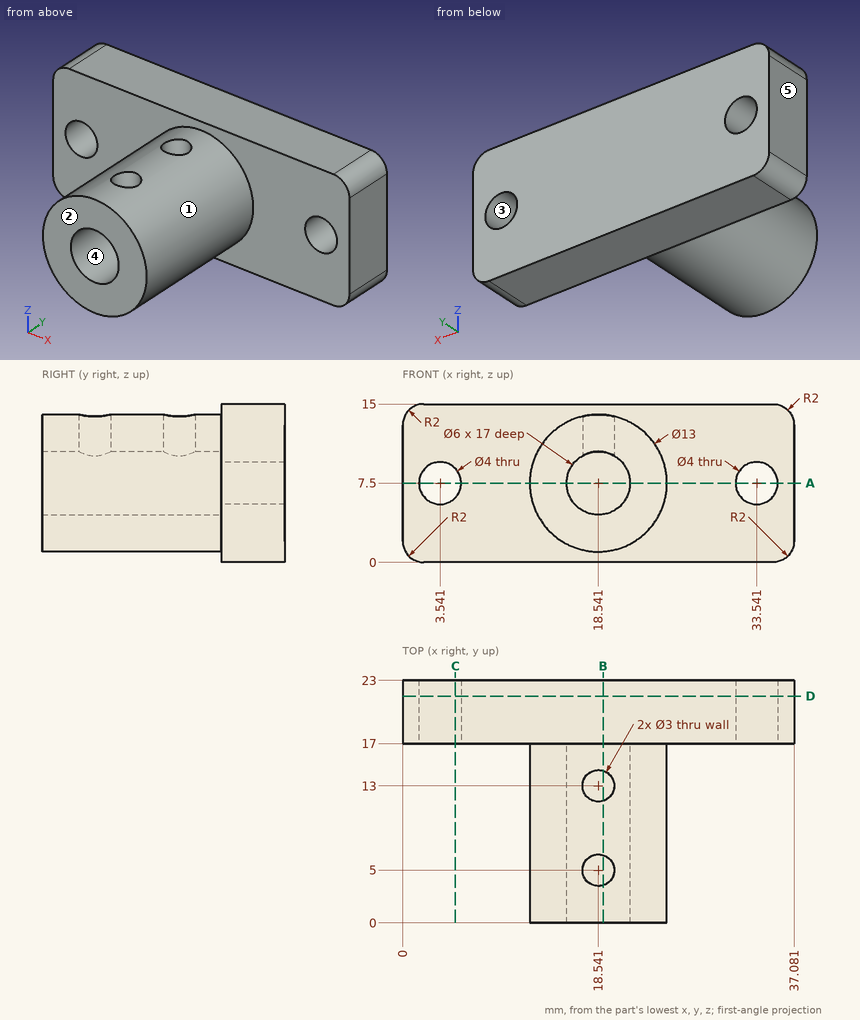
Design review of the part shown in the three views and the two pictorial views. Dimensions are in mm from the part's minimum x, y and z. A direction names the side the tool comes from. Give positions to 0.01 mm unless a question says otherwise; leave off trailing zeros. Order: outer loops, then holes, each group sorted by start corner. A loop starts at its lowest first (then second) coordinate and runs counter-clockwise, first axis right, second up. Notation, with made-up numbers: (53, 14) -> (97, 14) arc R21 ccw to (97, 29) -> close; hole circle Ø7 at (74, 33). An arc over 180 degrees is marked (long way). Write each question's results on one line, items separated by ' | '. Start each with the question number.
Q1. Add section C-C on x = 5. Give the boundary of the cut face in (y, z).
Q2. Add section B-B on x = 19. Give the boundary of the cut face in (y, z) (1 decimal).
Q3. Add section D-D on y = 21.5. Give the boundary of the cut face in (x, z).
Q4. Mouldability with a two-part tool opening along X and no side actions: class the marked faces 1, 2 and 3 as +X half, -X half, draft (parallel to the pull), parting line (faces both ways), or undercut.
Q5. Wall thickness on L1, parallel to X at y = 21, z = 7.5; L2, parallel to Y at x = 2.5, z = 4.25; L3, parallel to X at y = 13, z = 10.9: over which ranges is each line inside the solid? List them lowest first. Write a range as from..to.
Q6. Add section A-A on z = 7.5. Give the boundary of the cut face in (x, y).
Q7. For pin 1 (3.5 mm diameter, centred on x = 18.54, y = 13, fed in from +Z); pin 2 (6.5 mm diameter, centred on x = 19, z = 7.5, fed in from -Y); pin 3 (12 mm diameter, centred on x = 7, y = 4, fed in from +Z); pin 4 (1 mm diameter, centred on x = 10.5, y = 6.5, fed in from +Z), all flat-tipped, find the tip position at first contact; note any pin that passes through.
Q8. Machinability: for the marked faces 4 and 5, which of the approach directions +Z, -Z, +X, -X, +Y, -Y give a long, thin tool a straight path to every point of the face, cutting with its end or side? Answer none if there is none.
Found:
1) outline: (17, 0) -> (23, 0) -> (23, 6.13) -> (17, 6.13) -> close; (17, 8.87) -> (23, 8.87) -> (23, 15) -> (17, 15) -> close
2) outline: (0, 1) -> (17, 1) -> (17, 0) -> (23, 0) -> (23, 15) -> (17, 15) -> (17, 14) -> (14.4, 14) -> (14.4, 10.5) -> (17, 10.5) -> (17, 4.5) -> (0, 4.5) -> close; (0, 10.5) -> (3.6, 10.5) -> (3.6, 14) -> (0, 14) -> close; (6.4, 10.5) -> (11.6, 10.5) -> (11.6, 14) -> (6.4, 14) -> close
3) outline: (0, 2) arc R2 ccw to (2, 0) -> (35.08, 0) arc R2 ccw to (37.08, 2) -> (37.08, 13) arc R2 ccw to (35.08, 15) -> (2, 15) arc R2 ccw to (0, 13) -> close; hole circle Ø4 at (3.54, 7.5); hole circle Ø4 at (33.54, 7.5)
4) face 1: parting line | face 2: draft | face 3: undercut
5) L1: x = 0..1.54, 5.54..31.54, 35.54..37.08 | L2: y = 17..23 | L3: x = 13..17.04, 20.04..24.08
6) outline: (0, 17) -> (1.54, 17) -> (1.54, 23) -> (0, 23) -> close; (5.54, 17) -> (12.04, 17) -> (12.04, 0) -> (15.54, 0) -> (15.54, 17) -> (21.54, 17) -> (21.54, 0) -> (25.04, 0) -> (25.04, 17) -> (31.54, 17) -> (31.54, 23) -> (5.54, 23) -> close; (35.54, 17) -> (37.08, 17) -> (37.08, 23) -> (35.54, 23) -> close
7) pin 1: stops at z = 14 | pin 2: stops at y = 0 | pin 3: stops at z = 10.9 | pin 4: passes through
8) face 4: -Y | face 5: +Z, -Z, -X, +Y, -Y
